Autodesk Inventor part; units mm, degrees
ref_plane "YZ Plane" through (0, 0, 0) normal (1, 0, 0) x (0, 1, 0)
ref_plane "XZ Plane" through (0, 0, 0) normal (0, 1, 0) x (-1, 0, 0)
ref_plane "XY Plane" through (0, 0, 0) normal (0, 0, 1) x (1, 0, 0)
sketch "Boceto1" plane through (0, 0, 0) normal (0, 1, 0) x (-1, 0, 0)
  circle A0 centre (0, 0) radius 18
  circle A1 centre (0, 0) radius 9.75
  dimension "d0" = 36
  dimension "d1" = 19.5
extrude "Extrusión1" add sketch "Boceto1" along normal blind 1.5
sketch "Boceto2" plane through (0, 1.5, 0) normal (0, 1, 0) x (1, 0, 0)
  circle A0 centre (0, 0) radius 9.75
  circle A1 centre (0, 0) radius 13.25
  dimension "d4" = 26.5
extrude "Extrusión2" add sketch "Boceto2" along normal blind 5
sketch "Boceto3" plane through (0, 1.5, 0) normal (0, 1, 0) x (1, 0, 0)
  circle A0 centre (0, 0) radius 18
  line L0 (18, 0) -> (18, -4.85)
  line L1 (18, -4.85) -> (12.3305, -4.85)
  circle A1 centre (0, 0) radius 13.25
  line L2 (18, 0) -> (18, 4.85)
  line L3 (18, 4.85) -> (12.3305, 4.85)
  point P0 (17.3343, 4.85)
  point P1 (17.3343, -4.85)
  dimension "d7" = 4.85
  dimension "d8" = 4.85
extrude "Extrusión3" cut sketch "Boceto3" against normal through all contours A0 L1 A1 L3 picked at (14.5628, -2.7275)
sketch "Boceto4" plane through (0, 0, 0) normal (0, 0, 1) x (1, 0, 0)
  line L0 (9.75, 6.5) -> (9.75, 0)
  line L1 (13.25, 0) -> (13.25, 6.5)
  line L2 (13.25, 6.5) -> (9.75, 6.5)
  line L3 (11.5, 6.5) -> (9.75, 3.25)
  line L4 (9.75, 3.25) -> (11.5, 0)
  line L5 (17.3343, 0) -> (-18, 0)
  line L6 (11.5, 0) -> (13.25, 0)
  line L7 (11.5, 0) -> (9.75, 0)
  line L8 (9.75, 0) -> (9.75, 6.5)
  line L9 (9.75, 6.5) -> (11.5, 6.5)
  line L10 (13.25, 6.5) -> (-13.25, 6.5)
  point P0 (0, 0)
sketch3d "Boceto 3D1"
  arc A0 (9.75, 6.5, 0) -> (0, 6.5, 9.75) centre (0, 6.5, 0) ccw
  arc A1 (0, 6.5, 9.75) -> (-9.75, 6.5, 0) centre (0, 6.5, 0) ccw
  arc A2 (-9.75, 6.5, 0) -> (0, 6.5, -9.75) centre (0, 6.5, 0) ccw
  arc A3 (0, 6.5, -9.75) -> (9.75, 6.5, 0) centre (0, 6.5, 0) ccw
sweep "Barrido1" cut profiles "Boceto4" path "Boceto 3D1" contours L2 L3 L0 | L4 L5 L0
properties part number "Sujección_piezas_sonar"
Build history of the part. All positions in model axes, mm. A direction names the side the tool comes from. Give positions to 0.01 mm unless a question says otherwise; leave off trailing zeros. Loops run counter-clockwise (first coordinate to the right, second up) from the corner with the lowest first, then second, coordinate; pieces in that order, holes last. Notation, with made-up numbers: (-17, 61.5) -> (15, 61.5) arc R15 ccw to (15, 73.5) -> close; hole circle Ø2 at (-35.5, 84.5). An arc over 180 degrees is marked (long way). Answer in a Markdown table with one row per item.
Item 1: Mould opens along X. For faces 1 (the cylindrical face through (12.64, 4.02, -3.98)), 2 (the conical face through (9.625, 3.453, 2.137)), 3 (the flat face through (-4, 6.5, -11)) say: pulls with the +X half, pulls with the -X half, needs draft (parallel to the pull), parting line crosses it, or undercut.
Findings below:
| item | result |
|---|---|
| face 1 | parting line crosses it |
| face 2 | undercut |
| face 3 | needs draft |
Item 2: Probe line 1 along Y through (x, z) = (13.5, 9); line 2 along X through (y, z) = (3.5, 8.5); line 3 along Z through (x, y) = (-1.5, 3.25). List the from-to ranges inside material, lowest first. Write a range as [from, to].
Findings below:
| item | result |
|---|---|
| line 1 | y = [0, 1.5] |
| line 2 | x = [-10.16, -5.05], [5.05, 10.16] |
| line 3 | z = [-13.16, -9.63], [9.63, 13.16] |
Item 3: Slice it at C-C on y = 0.75. Write the cut outline in (x, z).
Findings below:
| item | result |
|---|---|
| outline | (12.33, -4.85) arc R13.25 ccw to (12.33, 4.85) -> (17.33, 4.85) arc R18 ccw (long way) to (17.33, -4.85) -> close; hole circle Ø22.19 at (0, 0) |
Item 4: Flat gauge pins, fed straight in: P1, Ø1, axis at x = -10.5, z = 2, coming from the +Y side; P2, Ø0.8, axis at x = 14, y = 0.5, coming from the +Z side; P3, Ø1.5, axis at y = 5.5, z = 9.5, coming from the +X side. Where does each tip first touch, or does it go through?
Findings below:
| item | result |
|---|---|
| P1 | stops at y = 5.92 |
| P2 | stops at z = 11.79 |
| P3 | stops at x = 9.95 |
Item 5: Tool access for faces 4 (the cylindrical face through (-17.985, 0.74, 0.723)), 5 (the flat face through (-11, 1.5, -8)), 6 (the flat face through (15, 1, 4.85)): list every direction of +Z, -Z, +X, -X, +Y, -Y with a clear straight run to the whole face (end or side of a thin tool).
Findings below:
| item | result |
|---|---|
| face 4 | +Y, -Y |
| face 5 | +Y |
| face 6 | +X, +Y, -Y |
Item 6: Slice it at A-A on x = 0. Write the cut outline in (y, z).
Findings below:
| item | result |
|---|---|
| outline | (0, -18) -> (1.5, -18) -> (1.5, -13.25) -> (6.5, -13.25) -> (6.5, -11.5) -> (3.25, -9.75) -> (0, -11.5) -> close; (0, 11.5) -> (3.25, 9.75) -> (6.5, 11.5) -> (6.5, 13.25) -> (1.5, 13.25) -> (1.5, 18) -> (0, 18) -> close |
Item 7: Slice it at D-D on z = 14.5. Write the cut outline in (x, y).
Findings below:
| item | result |
|---|---|
| outline | (-10.67, 0) -> (10.67, 0) -> (10.67, 1.5) -> (-10.67, 1.5) -> close |
Item 8: Slice it at B-B on z = 0. Write the cut outline in (x, y).
Findings below:
| item | result |
|---|---|
| outline | (-18, 0) -> (-11.5, 0) -> (-9.75, 3.25) -> (-11.5, 6.5) -> (-13.25, 6.5) -> (-13.25, 1.5) -> (-18, 1.5) -> close; (9.75, 3.25) -> (11.5, 0) -> (13.25, 0) -> (13.25, 6.5) -> (11.5, 6.5) -> close |
